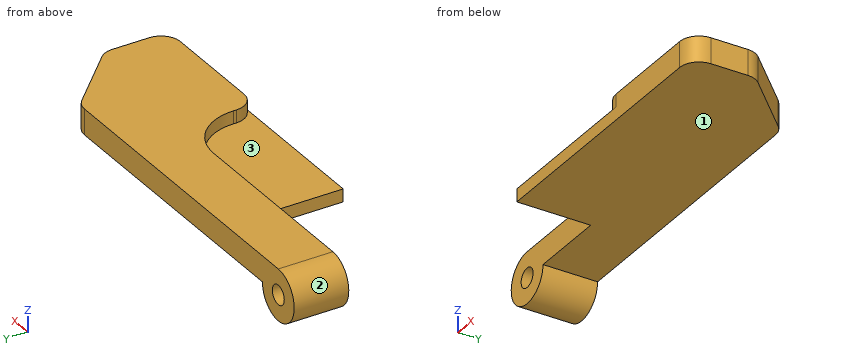
```python
from build123d import *

# Parameters (mm, degrees)
CROQUIS1_R              = 4
CROQUIS1_R_2            = 1.5
SALIENTE_EXTRUIR1_DEPTH = 20
CROQUIS2_W              = 27.807177066
CROQUIS2_H              = 11.5
CORTAR_EXTRUIR1_DEPTH   = 20
CROQUIS3_W              = 22
CROQUIS3_H              = 11.5
CORTAR_EXTRUIR2_DEPTH   = 2
CHAFL_N1_SIZE           = 10
REDONDEO1_R             = 3
REDONDEO2_R             = 3
REDONDEO3_R             = 3
REDONDEO4_R             = 8


with BuildPart() as part:
    # Croquis1 → Saliente-Extruir1 (new body)
    # profile 1 of 2: a face of its own
    with BuildSketch(Plane(origin=(0, 0, 0), x_dir=(1, 0, 0), z_dir=(0, 1, 0))):
        Circle(CROQUIS1_R)
        with Locations(Location((0, 0, 0), (0, 0, 270))):
            Circle(CROQUIS1_R_2, mode=Mode.SUBTRACT)
    # profile 2 of 2: a face of its own
    with BuildSketch(Plane(origin=(0, 0, 0), x_dir=(1, 0, 0), z_dir=(0, 1, 0))):
        with BuildLine():
            Line((60, 0), (4, 0))
            ThreePointArc((4, 0), (2.828427125, -2.828427125), (0, -4))
            Line((0, -4), (60, -4))
            Line((60, -4), (60, 0))
        make_face()
    extrude(amount=SALIENTE_EXTRUIR1_DEPTH)

    # Croquis2 → Cortar-Extruir1 (cut)
    with BuildSketch(Plane.XY.offset(4)):
        with Locations((2.096411467, 5.75)):
            Rectangle(CROQUIS2_W, CROQUIS2_H)
    extrude(amount=-CORTAR_EXTRUIR1_DEPTH, mode=Mode.SUBTRACT)

    # Croquis3 → Cortar-Extruir2 (cut)
    with BuildSketch(Plane.XY.offset(4)):
        with Locations((27, 5.75)):
            Rectangle(CROQUIS3_W, CROQUIS3_H)
    extrude(amount=-CORTAR_EXTRUIR2_DEPTH, mode=Mode.SUBTRACT)

    # Chaflán1
    chafl_n1_edges = [part.edges().sort_by_distance(p)[0] for p in [
        (60, 20, 2),
    ]]
    chamfer(chafl_n1_edges, length=CHAFL_N1_SIZE)

    # Redondeo1
    redondeo1_edges = [part.edges().sort_by_distance(p)[0] for p in [
        (60, 0, 2),
    ]]
    fillet(redondeo1_edges, radius=REDONDEO1_R)

    # Redondeo2
    redondeo2_edges = [part.edges().sort_by_distance(p)[0] for p in [
        (50, 20, 2),
        (60, 10, 2),
    ]]
    fillet(redondeo2_edges, radius=REDONDEO2_R)

    # Redondeo3
    redondeo3_edges = [part.edges().sort_by_distance(p)[0] for p in [
        (38, 0, 3),
    ]]
    fillet(redondeo3_edges, radius=REDONDEO3_R)

    # Redondeo4
    redondeo4_edges = [part.edges().sort_by_distance(p)[0] for p in [
        (38, 11.5, 3),
    ]]
    fillet(redondeo4_edges, radius=REDONDEO4_R)


solid = part.part
```
Check sheet for the modelled part. Datum: model origin and axes. Units: mm. Face numbers are marked on the shaded views. A direction names the side the tool comes from. Give positions to 0.01 mm unless a question says otherwise; leave off trailing zeros. Loops run counter-clockwise (first coordinate to the right, second up) from the corner with the lowest first, then second, coordinate; pieces in that order, holes last. Notation, with made-up numbers: (-37.5, 85) - (-31.5, 85) arc R25 ccw to (-31.5, 116) - close; hole circle Ø8 at (70.25, 36.5). An arc over 180 degrees is marked (long way). One line per question, with ' | ' between items. Start each with the question number.
1. Cross-section at A-A, the plane y = 12.75. Enter the section's corners in (x, z), plus the area to 3 significant figures.
2. Cross-section at D-D, the plane x = 23.5. Enter the section's corners in (y, z).
3. Cross-section at C-C, the plane z = -3. Enter the section's corners in (x, y), plus the area to 3 significant figures.
4. Set-up check for the marked faces 1, 2 and 3: record each of +Z, -Z, +X, -X, +Y, -Y from which the full face is reachable in a straight line by a thin tool's end or side.
5. Cross-section at B-B, the plane x = 44. Enter the section's corners in (y, z), plus the area to 3 significant figures.
6. Gauge pin test, flat ends, axial feed: pin 1 Ø1.5 at (x, y) = (16.5, 3.5) entering from -Z; pin 2 Ø3 at (x, z) = (39.5, -3) entering from -Y; pin 3 Ø0.6 at (y, z) = (5.5, 1) entering from -X; pin 4 Ø6 at (x, y) = (23.5, 7) entering from +Z. Record the tip position at first contact, or that the pin passes through.
7. Material ranges on line 1 along Z through (x, y) = (44, 15.25); line 2 along Y through (x, z) = (54, 0.75); line 3 along Z through (x, y) = (32.5, 8.25), recorded low to high. Write a range as [from, to].
Check result:
1) outline: (0, 4) arc R4 ccw (long way) to (4, 0) - (57.25, 0) - (57.25, 4) - close; hole circle Ø3 at (0, 0) | area: 260 mm2
2) outline: (0, 0) - (20, 0) - (20, 4) - (11.5, 4) - (11.5, 2) - (0, 2) - close
3) outline: (-2.65, 11.5) - (2.65, 11.5) - (2.65, 20) - (-2.65, 20) - close | area: 45.0 mm2
4) face 1: -Z, +X, +Y, -Y | face 2: +Y, -Y | face 3: +Z, -X, -Y
5) outline: (0, 0) - (20, 0) - (20, 4) - (0, 4) - close | area: 80.0 mm2
6) pin 1: stops at z = 0 | pin 2: passes through | pin 3: stops at x = 16 | pin 4: stops at z = 2
7) line 1: z = [0, 4] | line 2: y = [0, 16] | line 3: z = [0, 2]
